Solid Edge part; units mm, degrees
sketch "Sketch1" plane through (0, 0, 0) normal (0, 0, 1) x (1, 0, 0)
  circle A0 centre (0, 0) radius 10
extrude "Protrusion1" add sketch "Sketch1" along normal blind 5.5
sketch "Sketch2" plane through (0, 0, 0) normal (0, 0, -1) x (1, 0, 0)
  circle A0 centre (0, 0) radius 5
extrude "Protrusion2" add sketch "Sketch2" along normal blind 39.5
sketch "Sketch3" plane through (0, 0, -39.5) normal (0, 0, -1) x (1, 0, 0)
  circle A0 centre (0, 0) radius 4.9997
extrude "Cutout1" cut sketch "Sketch3" against normal blind 26 flip side to cut
chamfer "Chamfer_1" distance 0.75 angle 45 1 edges at (-4.9997, 0, -39.5)
sketch "Sketch4" plane through (0, 0, 5.5) normal (0, 0, 1) x (1, 0, 0)
  line L0 (-1.7321, 3) -> (1.7321, 3)
  line L1 (3.4641, 0) -> (1.7321, 3)
  line L2 (1.7321, -3) -> (3.4641, 0)
  line L3 (-1.7321, -3) -> (1.7321, -3)
  line L4 (-3.4641, 0) -> (-1.7321, -3)
  line L5 (-1.7321, 3) -> (-3.4641, 0)
extrude "Cutout2" cut sketch "Sketch4" against normal blind 3.6667
sketch "Sketch5" plane through (0, 0, 0) normal (0, -1, 0) x (1, 0, 0)
  line L0 (10, 5.5) -> (4.5, 0)
  line L1 (4.5, 0) -> (10, 0)
  line L2 (10, 0) -> (10, 5.5)
revolve "RevolvedCutout1" cut sketch "Sketch5" angle 360 about axis through (0, 0, 14.0017) along (0, 0, -1)
properties part number "185740" material "Stainless Steel, 304"
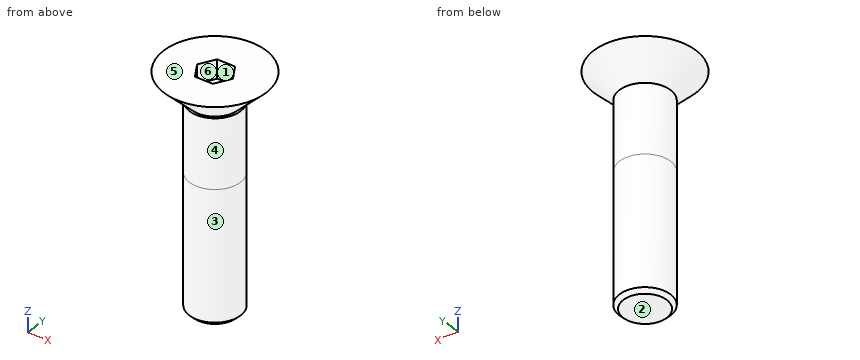
For this review, take the finished solid that the model builds, in its own axes (mm). Face numbers are marked on the shaded views. A direction names the side the tool comes from. Round coordinates to 2 decimals unless told otherwise and drop trailing zeros. Loops run counter-clockwise (first coordinate to the right, second up) from the corner with the lowest first, then second, coordinate; pieces in that order, holes last.
(1) Clearance check with flat-ended pins moving along their axes: P1, Ø1, axis at x = 0, z = 4, coming from the -Y side; P2, Ø1, axis at x = 1, y = 0, coming from the +Z side; P3, Ø4, axis at x = 2, z = -6, coming from the +Y side. State where each tip first meets the part, or that it passes through.
Returned:
P1: stops at y = -9
P2: stops at z = 1.83
P3: stops at y = 5
(2) Wall thickness on line 1 along Z through (x, y) = (-2.75, 4); line 2 along X through (y, z) = (4, -30.5); line 3 along X through (y, z) = (0, -12): over which ranges is each line inside the solid? List them lowest first.
Returned:
line 1: z = -38.9 to 0, 0.35 to 5.5
line 2: x = -3 to 3
line 3: x = -5 to 5
(3) Tool access review of the marked faces 1, 2 and 3: name each direction out of +Z, -Z, +X, -X, +Y, -Y from which nothing blocks a thin tool from reaching the whole face with its end or side.
Returned:
face 1: +Z
face 2: -Z, +X, -X, +Y, -Y
face 3: -Z
(4) We need section B-B (z = -14.5). Give the boundary of the cut face in (x, y).
Returned:
outline: circle Ø10 at (0, 0)
(5) Mouldability with a two-part tool opening along Y and no side actions: class the marked faces 4, 5 and 6 as released by +Y, released by -Y, zero draft, split by the parting line, or undercut.
Returned:
face 4: split by the parting line
face 5: zero draft
face 6: undercut
